```python
from build123d import *

# Parameters (mm, degrees)
F0_W      = 5
F0_H      = 5
F1_DEPTH  = 8.89
F2_W      = 14.4415530376
F2_H      = 5.6946645491
F3_DEPTH  = 12.7
F4_W      = 8.575418964
F4_H      = 1.1608570348
F4_H_2    = 5.6946645491
F5_DEPTH  = 6.35
F6_W      = 3.4819149878
F6_H      = 4.0748249739
F7_DEPTH  = 2.54
F8_W      = 4.1677881964
F8_H      = 3.9033070207
F9_DEPTH  = 2.54
F11_W     = 1.27
F11_H     = 3.4819149878
F10_W     = 1.27
F10_H     = 4.1677881964
F12_DEPTH = 2.54
F13_R     = 1.0279027568
F13_R_2   = 0.8784163787
F14_DEPTH = 0.762


with BuildPart() as f1:
    # F0 (on Top) → F1 (new body)
    with BuildSketch(Plane.XY):
        with Locations((-7.5847473372, 0)):
            Rectangle(F0_W, F0_H)
    extrude(amount=F1_DEPTH)



with BuildPart() as f1b:
    # F0 (on Top) → F1, piece 2 (new body)
    with BuildSketch(Plane.XY):
        with Locations((0.9745767244, 0)):
            Rectangle(F0_W, F0_H)
    extrude(amount=F1_DEPTH)


with BuildPart() as f1_1:
    add(f1.part)

    add(f1b.part)  # F3 merges F1b
    # F2 (on Top) → F3 (join)
    with BuildSketch(Plane.XY):
        with Locations((-3.1453159172, 0)):
            Rectangle(F2_W, F2_H)
    extrude(amount=-F3_DEPTH)

    # F4 (on face) → F5 (join)
    with BuildSketch(Plane(origin=(0, 0, -12.7), x_dir=(1, 0, 0), z_dir=(0, 0, -1))):
        with Locations((-3.1367521733, -3.427760792)):
            Rectangle(F4_W, F4_H)
        with Locations((-3.1367521733, 3.427760792)):
            Rectangle(F4_W, F4_H)
        with Locations((-3.1367521733, 0)):
            Rectangle(F4_W, F4_H_2)
    extrude(amount=F5_DEPTH)

    # F6 (on face) → F7 (join)
    with BuildSketch(Plane.YZ.offset(4.0754606016)):
        with Locations((0, -7.4885827489)):
            Rectangle(F6_W, F6_H)
    extrude(amount=F7_DEPTH)

    # F8 (on face) → F9 (join)
    with BuildSketch(Plane(origin=(-10.366092436, 0, 0), x_dir=(0, -1, 0), z_dir=(-1, 0, 0))):
        with Locations((0, -7.2363391519)):
            Rectangle(F8_W, F8_H)
    extrude(amount=F9_DEPTH)

    # F11 (on face) + F10 (on face) → F12 (join)
    with BuildSketch(Plane.XY.offset(-5.4511702619)):
        with Locations((5.9804606016, 0)):
            Rectangle(F11_W, F11_H)
    with BuildSketch(Plane.XY.offset(-5.2846856415)):
        with Locations((-12.271092436, 0)):
            Rectangle(F10_W, F10_H)
    extrude(amount=F12_DEPTH)

    # F13 (on face) → F14 (cut)
    with BuildSketch(Plane.XZ.offset(4.0081893094)):
        with Locations((-0.5419000518, -16.7948883027)):
            Circle(F13_R)
        with Locations((-5.2912211977, -16.5589284152)):
            Circle(F13_R_2)
        with BuildLine():
            add(Edge.make_bspline(
                [(-4.6211974695, -14.8275010288), (-4.6525107879, -14.3582631191), (-2.8178407576, -12.9321177777), (-0.316711825, -14.9404321969), (-1.9384263234, -15.4575665045), (-2.7810199858, -13.9257072681), (-3.7237353615, -15.5727199427), (-4.6015179058, -15.1224042148), (-4.6211974695, -14.8275010288)],
                knots=[0, 0, 0, 0, 0.2079480328, 0.4192374914, 0.5500370632, 0.7069707366, 0.8693103517, 1, 1, 1, 1], degree=3))
        make_face()
    extrude(amount=-F14_DEPTH, mode=Mode.SUBTRACT)


solid = f1_1.part
```
The listing builds one solid part. Answer for the finished solid, in the listing's coordinates (mm). A direction names the side the tool comes from. Coordinates: 2 decimals unless noted, no trailing zeros. Write each loop counter-clockwise with the first axis right and the second up, starting at its lowest first coordinate (ties: lowest second). Pieces come first, ordered by that corner, then holes.
Q1. Which of the six approach directions +Z, -Z, +X, -X, +Y, -Y give full straight-line access (tool end or side, diameter ignored) to faces 1 (the flat face through (-12, 2.084, -7)), 2 (the flat face through (-1.525, 0, 4)), 3 (the flat face through (3, 0, -12.7)), 4 (the flat face through (1, 2.5, 4)), 5 (the flat face through (-12, 0, -2.745))?
Returned:
face 1: +Z, -Z, -X, +Y
face 2: +Z, +Y, -Y
face 3: -Z, +X, +Y, -Y
face 4: +Z, +X, -X, +Y
face 5: +Z, -X, +Y, -Y
Q2. Given P1, Ø2, axis at x = -11.5, z = -5, coming from the -Y side; P2, Ø8, axis at x = -5, z = 2, coming from the +Y side; P3, Ø1.9, axis at y = 0.5, z = -17, coming from the +X side, each flat-ended and moving along its own axis, determine where each tip first touches the part or whether it passes through.
Returned:
P1: stops at y = -2.08
P2: stops at y = 2.85
P3: stops at x = 1.15
Q3. Section D-D, the plane z = -1 is taken. Write down the section's boundary in (x, y).
Returned:
outline: (-10.37, -2.85) - (4.08, -2.85) - (4.08, 2.85) - (-10.37, 2.85) - close
Q4. Section A-A, the plane z = 6.25 is taken. Write down the section's boundary in (x, y).
Returned:
outline: (-10.08, -2.5) - (-5.08, -2.5) - (-5.08, 2.5) - (-10.08, 2.5) - close; (-1.53, -2.5) - (3.47, -2.5) - (3.47, 2.5) - (-1.53, 2.5) - close
Q5. Section B-B, the plane y = 1 is taken. Write down the section's boundary in (x, z), then the cut area to 3 significant figures.
Returned:
outline: (-12.91, -9.19) - (-10.37, -9.19) - (-10.37, -12.7) - (-7.42, -12.7) - (-7.42, -19.05) - (1.15, -19.05) - (1.15, -12.7) - (4.08, -12.7) - (4.08, -9.53) - (6.62, -9.53) - (6.62, -2.91) - (5.35, -2.91) - (5.35, -5.45) - (4.08, -5.45) - (4.08, 0) - (3.47, 0) - (3.47, 8.89) - (-1.53, 8.89) - (-1.53, 0) - (-5.08, 0) - (-5.08, 8.89) - (-10.08, 8.89) - (-10.08, 0) - (-10.37, 0) - (-10.37, -5.28) - (-11.64, -5.28) - (-11.64, -2.74) - (-12.91, -2.74) - close
area: 353 mm2
Q6. The mould has two halves that part along X. Classify faces 6 (the flat face through (-8, 0, 8.89)), 7 (the flat face through (3.475, 0, 4)), 8 (the flat face through (-11.636, 0, -4)): released by +X, released by -X, zero draft, split by the parting line, or undercut.
Returned:
face 6: zero draft
face 7: released by +X
face 8: undercut
Q7. Find the intervals of material crossed by line 1 along X through (y, z) = (-1.75, 0.25); line 2 along X through (y, z) = (0.75, -16.25); line 3 along Z through (x, y) = (-10.5, 0.75), in increasing order.
Returned:
line 1: x = -10.08 to -5.08, -1.53 to 3.47
line 2: x = -7.42 to 1.15
line 3: z = -9.19 to -5.28
Q8. Section C-C, the plane x = 2.25 is taken. Write down the section's boundary in (y, z), then the cut area to 3 significant figures.
Returned:
outline: (-2.85, -12.7) - (2.85, -12.7) - (2.85, 0) - (2.5, 0) - (2.5, 8.89) - (-2.5, 8.89) - (-2.5, 0) - (-2.85, 0) - close
area: 117 mm2
